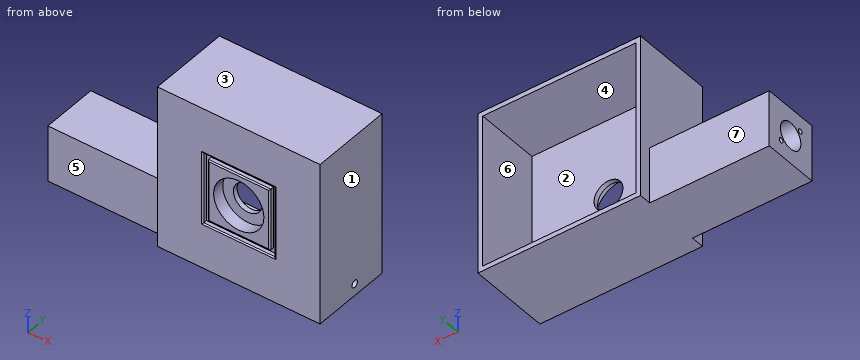
```python
from build123d import *

# Parameters (mm, degrees)
SKETCH1_W           = 68
SKETCH1_H           = 68
BOSS_EXTRUDE1_DEPTH = 34
CUT_EXTRUDE1_START  = 34
SKETCH2_W           = 64
SKETCH2_H           = 64
CUT_EXTRUDE1_DEPTH  = 27
SKETCH6_R           = 10.5
CUT_EXTRUDE10_DEPTH = 5
SKETCH7_W           = 30
SKETCH7_H           = 30
SKETCH7_W_2         = 26
SKETCH7_H_2         = 26
CUT_EXTRUDE11_DEPTH = 2
SKETCH8_R           = 1.5
CUT_EXTRUDE12_DEPTH = 3
SKETCH9_W           = 23.5
SKETCH9_H           = 23.5
SKETCH9_R           = 5.6
BOSS_EXTRUDE4_DEPTH = 50
SKETCH11_R          = 1
CUT_EXTRUDE13_DEPTH = 52
SKETCH5_R           = 6.05
CUT_EXTRUDE14_DEPTH = 35
FILLET1_R           = 0.5


with BuildPart() as part:
    # Sketch1 → Boss-Extrude1 (new body)
    with BuildSketch(Plane(origin=(0, 0, 0), x_dir=(1, 0, 0), z_dir=(0, 1, 0))):
        Rectangle(SKETCH1_W, SKETCH1_H)
    extrude(amount=BOSS_EXTRUDE1_DEPTH)

    # Sketch2 → Cut-Extrude1 (cut)
    with BuildSketch(Plane(origin=(0, 0, 0), x_dir=(1, 0, 0), z_dir=(0, 1, 0)).offset(CUT_EXTRUDE1_START)):
        Rectangle(SKETCH2_W, SKETCH2_H)
    extrude(amount=-CUT_EXTRUDE1_DEPTH, mode=Mode.SUBTRACT)

    # Sketch6 → Cut-Extrude10 (cut)
    with BuildSketch(Plane.XZ):
        Circle(SKETCH6_R)
    extrude(amount=-CUT_EXTRUDE10_DEPTH, mode=Mode.SUBTRACT)

    # Sketch7 → Cut-Extrude11 (cut)
    with BuildSketch(Plane(origin=(0, 0, 0), x_dir=(-1, 0, 0), z_dir=(0, -1, 0))):
        Rectangle(SKETCH7_W, SKETCH7_H)
        Rectangle(SKETCH7_W_2, SKETCH7_H_2, mode=Mode.SUBTRACT)
    extrude(amount=-CUT_EXTRUDE11_DEPTH, mode=Mode.SUBTRACT)

    # Sketch8 → Cut-Extrude12 (cut, through all)
    with BuildSketch(Plane.ZY.offset(-32)):
        with Locations((-29, 19)):
            Circle(SKETCH8_R)
    extrude(amount=-CUT_EXTRUDE12_DEPTH, mode=Mode.SUBTRACT)

    # Sketch9 → Boss-Extrude4 (add)
    with BuildSketch(Plane.ZY.offset(34)):
        with Locations((-22.25, 17.25)):
            Rectangle(SKETCH9_W, SKETCH9_H)
        with Locations((-22.25, 17.25)):
            Circle(SKETCH9_R, mode=Mode.SUBTRACT)
    extrude(amount=BOSS_EXTRUDE4_DEPTH)

    # Sketch11 → Cut-Extrude13 (cut)
    with BuildSketch(Plane.ZY.offset(84)):
        with Locations((-27.482590181, 22.482590181)):
            Circle(SKETCH11_R)
        with Locations((-17.017409819, 12.017409819)):
            Circle(SKETCH11_R)
    extrude(amount=-CUT_EXTRUDE13_DEPTH, mode=Mode.SUBTRACT)

    # Sketch5 → Cut-Extrude14 (cut, through all)
    with BuildSketch(Plane(origin=(0, 0, 0), x_dir=(1, 0, 0), z_dir=(0, 1, 0))):
        Circle(SKETCH5_R)
    extrude(amount=CUT_EXTRUDE14_DEPTH, mode=Mode.SUBTRACT)

    # Fillet1
    fillet1_edges = [part.edges().sort_by_distance(p)[0] for p in [
        (15, 0, 0),
        (0, 0, 15),
        (-15, 0, 0),
        (0, 0, -15),
        (13, 0, 0),
        (0, 0, -13),
        (-13, 0, 0),
        (0, 0, 13),
    ]]
    fillet(fillet1_edges, radius=FILLET1_R)


solid = part.part
```
For this review, take the finished solid that the model builds, in its own axes (mm). Face numbers are marked on the shaded views. A direction names the side the tool comes from. Coordinates: 2 decimals unless noted, no trailing zeros. Order: outer loops, then holes, each group sorted by start corner. A loop starts at its lowest first (then second) coordinate and runs counter-clockwise, first axis right, second up. Notation, with made-up numbers: (-15, 14) - (33, 14) arc R13 ccw to (33, 34) - close; hole circle Ø7 at (12, 66). An arc over 180 degrees is marked (long way). Answer as a JSON object with one key per item and string values. Group by question number.
1. The part is to be moulded in two halves that separate along X. For the marked faces 1, 2, 3 and 4, say which applies: pulls with the +X half, pulls with the -X half, needs draft (parallel to the pull), parting line crosses it, or undercut.
2. Clearance check with flat-ended pins moving along their axes: P1, Ø17, axis at x = 0, z = 0, coming from the +Y side; P2, Ø17, axis at y = 21, z = 3.5, coming from the -X side; P3, Ø10.5, axis at x = -3.5, z = -3.5, coming from the -Y side. State where each tip first meets the part, or that it passes through.
3. We need section D-D on x = -19.5. State the section outline as (y, z) points.
4. We need section B-B on z = 0. State the section outline as (x, y) points.
5. We need section A-A on x = 0. State the section outline as (y, z) points.
6. For the marked faces 5, 6 and 7, list the 3-axis set-ups (+Z, -Z, +X, -X, +Y, -Y) from which the entire face can be reached by the end or side of a thin tool; tool diameter is ignored.
7. For probe 1 along X at (y, z) = (13, 14.5); probe 2 along X at (y, z) = (8.5, -16), list the stretches that pass through material, from the lowest coordinate up.
8. We need section C-C on y = 9. State the section outline as (x, z) points, then the cut area to 3 significant figures.
Final values:
{
 "1": {"face 1": "pulls with the +X half", "face 2": "undercut", "face 3": "needs draft", "face 4": "undercut"},
 "2": {"P1": "y = 7", "P2": "x = -34", "P3": "y = 5"},
 "3": {"outline": "(0, -34) - (34, -34) - (34, -32) - (7, -32) - (7, 32) - (34, 32) - (34, 34) - (0, 34) - close"},
 "4": {"outline": "(-34, 0) - (-15.5, 0) arc R0.5 ccw to (-15, 0.5) - (-15, 2) - (-13, 2) - (-13, 0.5) arc R0.5 ccw to (-12.5, 0) - (-10.5, 0) - (-10.5, 5) - (-6.05, 5) - (-6.05, 7) - (-32, 7) - (-32, 34) - (-34, 34) - close; (6.05, 5) - (10.5, 5) - (10.5, 0) - (12.5, 0) arc R0.5 ccw to (13, 0.5) - (13, 2) - (15, 2) - (15, 0.5) arc R0.5 ccw to (15.5, 0) - (34, 0) - (34, 34) - (32, 34) - (32, 7) - (6.05, 7) - close"},
 "5": {"outline": "(0, -34) - (34, -34) - (34, -32) - (7, -32) - (7, -6.05) - (5, -6.05) - (5, -10.5) - (0, -10.5) - (0, -12.5) arc R0.5 ccw to (0.5, -13) - (2, -13) - (2, -15) - (0.5, -15) arc R0.5 ccw to (0, -15.5) - close; (0, 10.5) - (5, 10.5) - (5, 6.05) - (7, 6.05) - (7, 32) - (34, 32) - (34, 34) - (0, 34) - (0, 15.5) arc R0.5 ccw to (0.5, 15) - (2, 15) - (2, 13) - (0.5, 13) arc R0.5 ccw to (0, 12.5) - close"},
 "6": {"face 5": "+Z, -Z, -X, -Y", "face 6": "+Y", "face 7": "+Z, -Z, -X, +Y"},
 "7": {"probe 1": "-34 to -32, 32 to 34", "probe 2": "-84 to -32, 32 to 34"},
 "8": {"outline": "(-84, -34) - (34, -34) - (34, 34) - (-34, 34) - (-34, -10.5) - (-84, -10.5) - close; hole (-32, -32) - (32, -32) - (32, 32) - (-32, 32) - close", "area": "1,700 mm²"}
}
